from build123d import *

# Parameters (mm, degrees)
SKETCH1_R                      = 1.98501
BASE_EXTRUDE_DEPTH             = 9.525
SKETCH2_R                      = 1.98501
SKETCH2_R_2                    = 1.5621
CUT_EXTRUDE2_DEPTH             = 3.9624
CHAMFER1_SIZE                  = 0.254
CHAMFER2_SIZE                  = 0.762
SKETCH4_R                      = 0.1905
F_1_16_0_0625_DIAMETER_HOLE1_D = 1.5875


with BuildPart() as part:
    # Sketch1 → Base-Extrude (new body)
    with BuildSketch(Plane(origin=(0, 0, 0), x_dir=(1, 0, 0), z_dir=(0, 1, 0))):
        with Locations(Location((0, 0, 0), (0, 0, 270))):  # turned: the seam where the file's is
            Circle(SKETCH1_R)
    extrude(amount=BASE_EXTRUDE_DEPTH)

    # Sketch2 → Cut-Extrude2 (cut)
    with BuildSketch(Plane(origin=(0, 9.525, 0), x_dir=(1, 0, 0), z_dir=(0, 1, 0))):
        with Locations(Location((0, 0, 0), (0, 0, 270))):  # turned: the seam where the file's is
            Circle(SKETCH2_R)
        with Locations(Location((0, 0, 0), (0, 0, 270))):  # turned: the seam where the file's is
            Circle(SKETCH2_R_2, mode=Mode.SUBTRACT)
    extrude(amount=-CUT_EXTRUDE2_DEPTH, mode=Mode.SUBTRACT)

    # Chamfer1
    chamfer1_edges = [part.edges().sort_by_distance(p)[0] for p in [
        (0, 9.525, -1.5621),
    ]]
    chamfer(chamfer1_edges, length=CHAMFER1_SIZE)

    # Chamfer2
    chamfer2_edges = [part.edges().sort_by_distance(p)[0] for p in [
        (0, 0, -1.98501),
    ]]
    chamfer(chamfer2_edges, length=CHAMFER2_SIZE)

    # Sketch4 → Cut-Revolve1 (revolve, cut)
    with BuildSketch(Plane.XY, mode=Mode.PRIVATE) as cut_revolve1_sk:
        with Locations((-1.5621, 5.7531)):
            Circle(SKETCH4_R)
    revolve(cut_revolve1_sk.sketch.rotate(Axis((0, 9.525, 0), (0, -1, 0)), 270), axis=Axis((0, 9.525, 0), (0, -1, 0)), mode=Mode.SUBTRACT)  # turned: the seam where the file's is

    # 1/16 (0.0625) Diameter Hole1 (through all)
    with Locations(Plane(origin=(0, 9.525, 0), x_dir=(-1, 0, 0), z_dir=(0, 1, 0))):
        with Locations((0, 0)):
            Hole(F_1_16_0_0625_DIAMETER_HOLE1_D / 2)


solid = part.part
Design review of the part built by this model. Coordinates are the model's own, in mm. Coordinates: 2 decimals unless noted, no trailing zeros. Loops run counter-clockwise (first coordinate to the right, second up) from the corner with the lowest first, then second, coordinate; pieces in that order, holes last. Notation, with made-up numbers: (-8, 54) -> (44, 54) arc R21 ccw to (44, 60) -> close; hole circle Ø3 at (89.5, -15.5). An arc over 180 degrees is marked (long way). Use a Markdown table: item, result. Add a question column.
Item 1: Wall thickness on L1, parallel to X at y = 2, z = 0.3; L2, parallel to Z at x = -1.35, y = 7.75; L3, parallel to X at y = 6.5, z = 1.3: over which ranges is each line inside the solid? List them lowest first. Write a range as from..to.
Item 2: Clearance check with flat-ended pins moving along their axes: P1, Ø1.2, axis at x = 0, z = 0, coming from the +Y side; P2, Ø1.5, axis at x = -1.5, y = 4.5, coming from the -Z side. State where each tip first meets the part, or that it passes through.
Item 3: We need section C-C, the plane y = 2.5. Write out the cut boundary in (x, z), and give its area (3 significant figures).
Item 4: The part is to be moulded in two halves that separate along Z. For faces 1 (the cylindrical face through (-0.172, 4.696, -0.775)), 2 (the cylindrical face through (0.47, 7.63, 1.49)), 3 (the flat face through (0, 0, 1)), say which applies: +Z half, -Z half, draft (parallel to the pull), parting line (faces both ways), or undercut.
Numbers:
| question | item | result |
|---|---|---|
| 1 | L1 | x = -1.96..-0.73, 0.73..1.96 |
| 1 | L2 | z = -0.79..0.79 |
| 1 | L3 | x = -0.87..0.87 |
| 2 | P1 | passes through |
| 2 | P2 | stops at z = -1.84 |
| 3 | outline | circle Ø3.97 at (0, 0); hole circle Ø1.59 at (0, 0) |
| 3 | area | 10.4 mm^2 |
| 4 | face 1 | undercut |
| 4 | face 2 | parting line |
| 4 | face 3 | draft |
